Read the model definition and answer for the solid it produces. Units are mm, in the model's axes. Face numbers are marked on the shaded views. A direction names the side the tool comes from. Give positions to 0.01 mm unless a question says otherwise; leave off trailing zeros. Loops run counter-clockwise (first coordinate to the right, second up) from the corner with the lowest first, then second, coordinate; pieces in that order, holes last. Notation, with made-up numbers: (-38, 37) - (-6, 37) arc R16 cw to (-6, 61) - close; hole circle Ø1 at (-37, 72.25). An arc over 180 degrees is marked (long way). Put each result on its own line as item: value. Start each with the question number.
1. A cutting plane is placed at D-D, the plane x = 8.75. Determine the outline of the cut face in (y, z), plus the area to 3 significant figures.
2. For the marked faces 1, 2 and 3, determine the directions among +Z, -Z, +X, -X, +Y, -Y from which every point of the face is accessible in a straight line to the end or side of a thin tool.
3. For a pull along Z with two mould halves and no side action, classify the marked faces 4, 5, 6 and 7 as released by +Z, released by -Z, zero draft, split by the parting line, or undercut.
4. A cutting plane is placed at C-C, the plane z = 15. Determine the outline of the cut face in (x, y).
5. Given pin 1 Ø8 at (y, z) = (8.5, 7) entering from -X; pin 2 Ø1 at (x, z) = (26.5, 11.5) entering from -Y; pin 3 Ø4 at (x, z) = (16, 10.5) entering from +Y, each flat-ended and moving along its own axis, determine where each tip first touches the part or whether it passes through.
6. A cutting plane is placed at A-A, the plane x = 5. Count the separate pieces of the cut face and the enclosed holes in it, plus the area to 3 significant figures.
7. Consider L1, parallel to X at y = -5, z = 19.3; L2, parallel to Z at x = 5.75, y = 34; L3, parallel to Y at x = 25, z = 20.15. Determine where each line is inside the solid, lowest interval first. Write a range as from..to.
8. A cutting plane is placed at B-B, the plane y = -5. Determine the outline of the cut face in (x, z), plus the area to 3 significant figures.
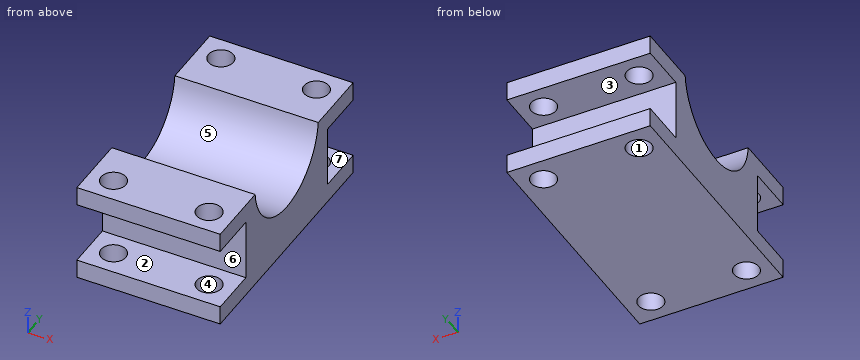
```python
from build123d import *

# Parameters (mm, degrees)
SKETCH_1_W          = 30
SKETCH_1_H          = 32
EXTRUDE_1_DEPTH     = 7
EXTRUDE_2_DEPTH     = 30
SKETCH_3_R          = 2.6
EXTRUDE_3_DEPTH     = 4
SKETCH_4_W          = 30
SKETCH_4_H          = 4
EXTRUDE_5_DEPTH     = 10
SKETCH_5_W          = 30
SKETCH_5_H          = 4
EXTRUDE_6_DEPTH     = 10
CUT_EXTRUDE_START   = -10
SKETCH_6_R          = 2.6
CUT_EXTRUDE_1_DEPTH = 10


with BuildPart() as part:
    # Эскиз1 → Бобышка-Вытянуть1 (new body)
    with BuildSketch(Plane.XY):
        with Locations((15, 16)):
            Rectangle(SKETCH_1_W, SKETCH_1_H)
    extrude(amount=EXTRUDE_1_DEPTH)

    # Эскиз2 → Бобышка-Вытянуть2 (add)
    with BuildSketch(Plane.ZY):
        with BuildLine():
            Line((7, 32), (20.887570227, 32))
            Line((20.887570227, 32), (20.887570227, 28.35))
            ThreePointArc((20.887570227, 28.35), (9.6, 16), (20.887570227, 3.65))
            Line((20.887570227, 3.65), (20.887570227, 0))
            Line((20.887570227, 0), (7, 0))
            Line((7, 0), (7, 32))
        make_face()
    extrude(amount=-EXTRUDE_2_DEPTH)

    # Эскиз3 → Бобышка-Вытянуть3 (add)
    with BuildSketch(Plane(origin=(0, 0, 0), x_dir=(-1, 0, 0), z_dir=(0, 0, -1))):
        Polygon((-30, 16), (-30, -10), (0, -10), (0, 42), (-30, 42), align=None)
        with Locations((-25, 37)):
            Circle(SKETCH_3_R, mode=Mode.SUBTRACT)
        with Locations((-5, 37)):
            Circle(SKETCH_3_R, mode=Mode.SUBTRACT)
        with Locations((-5, -5)):
            Circle(SKETCH_3_R, mode=Mode.SUBTRACT)
        with Locations((-25, -5)):
            Circle(SKETCH_3_R, mode=Mode.SUBTRACT)
    extrude(amount=-EXTRUDE_3_DEPTH)

    # Эскиз4 → Бобышка-Вытянуть5 (add)
    with BuildSketch(Plane(origin=(0, 32, 0), x_dir=(1, 0, 0), z_dir=(0, 1, 0))):
        with Locations((15, -18.887570227)):
            Rectangle(SKETCH_4_W, SKETCH_4_H)
    extrude(amount=EXTRUDE_5_DEPTH)

    # Эскиз5 → Бобышка-Вытянуть6 (add)
    with BuildSketch(Plane.XZ):
        with Locations((15, 18.887570227)):
            Rectangle(SKETCH_5_W, SKETCH_5_H)
    extrude(amount=EXTRUDE_6_DEPTH)

    # Эскиз6 → Вырез-Вытянуть1 (cut)
    with BuildSketch(Plane.XY.offset(20.887570227).offset(CUT_EXTRUDE_START)):
        with Locations(Location((5, 37, 0), (0, 0, 180))):
            Circle(SKETCH_6_R)
        with Locations(Location((25, 37, 0), (0, 0, 180))):
            Circle(SKETCH_6_R)
        with Locations(Location((25, -5, 0), (0, 0, 180))):
            Circle(SKETCH_6_R)
        with Locations(Location((5, -5, 0), (0, 0, 180))):
            Circle(SKETCH_6_R)
    extrude(amount=CUT_EXTRUDE_1_DEPTH, mode=Mode.SUBTRACT)


solid = part.part
```
Return value:
1. outline: (-10, 0) - (42, 0) - (42, 4) - (32, 4) - (32, 16.89) - (42, 16.89) - (42, 20.89) - (28.35, 20.89) arc R12.4 cw to (3.65, 20.89) - (-10, 20.89) - (-10, 16.89) - (0, 16.89) - (0, 4) - (-10, 4) - close
1. area: 614 mm2
2. face 1: +Z, -Z
2. face 2: +X, -X, -Y
2. face 3: +X, -X, +Y
3. face 4: zero draft
3. face 5: released by +Z
3. face 6: undercut
3. face 7: undercut
4. outline: (0, 0) - (30, 0) - (30, 5.76) - (0, 5.76) - close; (0, 26.24) - (30, 26.24) - (30, 32) - (0, 32) - close
5. pin 1: stops at x = 0
5. pin 2: stops at y = 0
5. pin 3: stops at y = 32
6. separate pieces: 5
6. enclosed holes: 0
6. area: 531 mm2
7. L1: x = 0..2.4, 7.6..22.4, 27.6..30
7. L2: z = 0..4, 16.89..20.89
7. L3: y = -10..-7.6, -2.4..3.74, 28.26..34.4, 39.6..42
8. outline: (0, 0) - (2.4, 0) - (2.4, 4) - (0, 4) - close; (0, 16.89) - (2.4, 16.89) - (2.4, 20.89) - (0, 20.89) - close; (7.6, 0) - (22.4, 0) - (22.4, 4) - (7.6, 4) - close; (7.6, 16.89) - (22.4, 16.89) - (22.4, 20.89) - (7.6, 20.89) - close; (27.6, 0) - (30, 0) - (30, 4) - (27.6, 4) - close; (27.6, 16.89) - (30, 16.89) - (30, 20.89) - (27.6, 20.89) - close
8. area: 157 mm2
